Build history of the part. All positions in model axes, mm. A direction names the side the tool comes from. Give positions to 0.01 mm unless a question says otherwise; leave off trailing zeros. Order: outer loops, then holes, each group sorted by start corner. A loop starts at its lowest first (then second) coordinate and runs counter-clockwise, first axis right, second up. Notation, with made-up numbers: (88.5, -8.5) -> (93.5, -8.5) arc R26 ccw to (93.5, 12.5) -> close; hole circle Ø7 at (88.25, -39.75). An arc over 180 degrees is marked (long way). Use a Markdown table: item, result. Add a question column.
```python
from build123d import *
from build123d.topology import SkipClean

# Parameters (mm, degrees)
ESQUISSE1_W             = 30
ESQUISSE1_H             = 6
ENL_V_MAT_EXTRU_4_DEPTH = 7.5
ENL_V_MAT_EXTRU_5_DEPTH = 15
ESQUISSE3_R             = 4.5
ENL_V_MAT_EXTRU_6_DEPTH = 10
ENL_V_MAT_EXTRU_9_DEPTH = 5


with BuildPart() as part:
    # Esquisse1 → Révolution1 (revolve)
    with BuildSketch(Plane(origin=(0, 0, 0), x_dir=(0, 0, -1), z_dir=(1, 0, 0)), mode=Mode.PRIVATE) as r_volution1_sk:
        with Locations((15, -3)):
            Rectangle(ESQUISSE1_W, ESQUISSE1_H)
    revolve(r_volution1_sk.sketch.rotate(Axis((0, 0, -30), (0, 0, 1)), 180), axis=Axis((0, 0, -30), (0, 0, 1)))

    # Esquisse2 → Enlèv. mat.-Extru.4 (cut)
    with BuildSketch(Plane.XY):
        with BuildLine():
            Line((-1.841364983, 1.5), (0, 1.5))
            Line((0, 1.5), (1.841364983, 1.5))
            ThreePointArc((1.841364983, 1.5), (0, 2.375), (-1.841364983, 1.5))
        make_face()
    extrude(amount=-ENL_V_MAT_EXTRU_4_DEPTH, mode=Mode.SUBTRACT)

    # Esquisse5 → Enlèv. mat.-Extru.5 (cut)
    with SkipClean():  # the faces are left unmerged after this step: merging them gives an invalid solid
        with BuildSketch(Plane.XY):
            with BuildLine():
                Line((-1.841364983, 1.5), (1.841364983, 1.5))
                ThreePointArc((1.841364983, 1.5), (0, -2.375), (-1.841364983, 1.5))
            make_face()
        extrude(amount=-ENL_V_MAT_EXTRU_5_DEPTH, mode=Mode.SUBTRACT)

    # Esquisse3 → Enlèv. mat.-Extru.6 (cut)
    with SkipClean():  # the faces are left unmerged after this step: merging them gives an invalid solid
        with BuildSketch(Plane(origin=(0, 0, -30), x_dir=(-1, 0, 0), z_dir=(0, 0, -1))):
            with Locations(Location((0, 0, 0), (0, 0, 90))):
                Circle(ESQUISSE3_R)
        extrude(amount=-ENL_V_MAT_EXTRU_6_DEPTH, mode=Mode.SUBTRACT)

    # Esquisse7 → Enlèv. mat.-Extru.9 (cut)
    with SkipClean():  # the faces are left unmerged after this step: merging them gives an invalid solid
        with BuildSketch(Plane(origin=(0, 0, -20), x_dir=(-1, 0, 0), z_dir=(0, 0, -1))):
            with BuildLine():
                Line((0, 2.5), (3.741657387, 2.5))
                ThreePointArc((3.741657387, 2.5), (0, -4.5), (-3.741657387, 2.5))
                Line((-3.741657387, 2.5), (0, 2.5))
            make_face()
        extrude(amount=-ENL_V_MAT_EXTRU_9_DEPTH, mode=Mode.SUBTRACT)


solid = part.part
```
(1) Pin check, flat tips, straight feed: pin 1 Ø4.5 at (x, y) = (0, 0) entering from +Z; pin 2 Ø1 at (x, z) = (2, -23) entering from +Y; pin 3 Ø4 at (x, y) = (0, 1) entering from -Z. Stop position of each tip, or through.
(2) Band-saw the part on C-C on z = -17.5. Give the cut face in (x, y).
(3) Mould opens along Y. For faces 5 (the face through (-1.802, 5.723, -15.21)), 6 (the face through (0, 2.5, -18)), 7 (the face through (-4.5, -1.4, -30)) say: released by +Y, released by -Y, zero draft, split by the parting line, or undercut.
(4) Wall check: probe 1 along X at (y, z) = (0, -26.25); probe 2 along X at (y, z) = (0, -7.75) (3 decimals); probe 3 along Y at (x, z) = (2, -17.75). Give the ranges that are in metal, low to high.
(5) Tool access for faces 1 (the face through (0, 3, 0)), 2 (the face through (0, 2, -7.5)), 3 (the face through (0, 1.5, -11)), 4 (the face through (0, 3, -20)): list every direction of +Z, -Z, +X, -X, +Y, -Y with a clear straight run to the whole face (end or side of a thin tool).
(6) Band-saw the part on B-B on y = 0. Give the cut face in (x, z) (3 decimals).
(7) Band-saw the part on D-D on x = -3. Give the cut face in (y, z).
(8) Band-saw the part on A-A on x = 0. Give the cut face in (y, z) (3 decimals), plus the area to 3 significant figures.
Response:
| question | item | result |
|---|---|---|
| 1 | pin 1 | stops at z = -7.5 |
| 1 | pin 2 | stops at y = 5.81 |
| 1 | pin 3 | stops at z = -20 |
| 2 | outline | circle Ø12 at (0, 0); hole (-3.74, 2.5) arc R4.5 ccw (long way) to (3.74, 2.5) -> close |
| 3 | face 5 | split by the parting line |
| 3 | face 6 | undercut |
| 3 | face 7 | zero draft |
| 4 | probe 1 | x = -6 to -4.5, 4.5 to 6 |
| 4 | probe 2 | x = -6 to -2.375, 2.375 to 6 |
| 4 | probe 3 | y = -5.66 to -4.03, 2.5 to 5.66 |
| 5 | face 1 | +Z, +X, -X, +Y, -Y |
| 5 | face 2 | +Z |
| 5 | face 3 | +Z, -Z |
| 5 | face 4 | -Z |
| 6 | outline | (-6, -30) -> (-4.5, -30) -> (-4.5, -15) -> (-2.375, -15) -> (-2.375, 0) -> (-6, 0) -> close; (2.375, -15) -> (4.5, -15) -> (4.5, -30) -> (6, -30) -> (6, 0) -> (2.375, 0) -> close |
| 7 | outline | (-5.2, -30) -> (-3.35, -30) -> (-3.35, -15) -> (2.5, -15) -> (2.5, -20) -> (3.35, -20) -> (3.35, -30) -> (5.2, -30) -> (5.2, 0) -> (-5.2, 0) -> close |
| 8 | outline | (-6, -30) -> (-4.5, -30) -> (-4.5, -15) -> (-2.375, -15) -> (-2.375, 0) -> (-6, 0) -> close; (1.5, -15) -> (2.5, -15) -> (2.5, -20) -> (4.5, -20) -> (4.5, -30) -> (6, -30) -> (6, 0) -> (2.375, 0) -> (2.375, -7.5) -> (1.5, -7.5) -> close |
| 8 | area | 170 mm² |
